```python
from build123d import *

# Parameters (mm, degrees)
BOSS_EXTRUDE1_DEPTH  = 7
BOSS_EXTRUDE2_DEPTH  = 60.3
SKETCH1_5_W          = 63.3
SKETCH1_5_H          = 5
BOSS_EXTRUDE3_DEPTH  = 60.3
SKETCH2_R            = 2.65
SKETCH2_R_2          = 3.5
CUT_EXTRUDE1_DEPTH   = 5
SKETCH2_3_R          = 19.05
CUT_EXTRUDE2_DEPTH   = 1.6
CUT_EXTRUDE3_DEPTH   = 5
BOSS_EXTRUDE6_DEPTH  = 5
BOSS_EXTRUDE10_DEPTH = 5
SKETCH15_R           = 3
SKETCH15_R_2         = 2
CUT_EXTRUDE7_DEPTH   = 5
SKETCH16_R           = 10
CUT_EXTRUDE8_DEPTH   = 5
SKETCH27_W           = 25
SKETCH27_H           = 87.5
CUT_EXTRUDE10_DEPTH  = 7
SKETCH33_R           = 3.5
BOSS_EXTRUDE18_DEPTH = 20


with BuildPart() as part:
    # Sketch1 → Boss-Extrude1 (new body)
    with BuildSketch(Plane(origin=(0, 0, 0), x_dir=(1, 0, 0), z_dir=(0, 1, 0))):
        Polygon((-1.592164976, 82.5), (61.707835024, 82.5), (86.707835024, 82.5), (86.707835024, -5), (61.707835024, -5), (-1.592164976, -5), (-26.592164976, -5), (-26.592164976, 82.5), align=None)
    extrude(amount=-BOSS_EXTRUDE1_DEPTH)

    # Sketch1<3> → Boss-Extrude2 (add)
    with BuildSketch(Plane(origin=(0, 0, 0), x_dir=(1, 0, 0), z_dir=(0, 1, 0))):
        Polygon((1.407835024, 0), (58.707835024, 0), (61.707835024, 0), (61.707835024, -5), (-1.592164976, -5), (-1.592164976, 0), align=None)
    extrude(amount=BOSS_EXTRUDE2_DEPTH)

    # Sketch1<5> → Boss-Extrude3 (add)
    with BuildSketch(Plane(origin=(0, 0, 0), x_dir=(1, 0, 0), z_dir=(0, 1, 0))):
        with Locations((30.057835024, 80)):
            Rectangle(SKETCH1_5_W, SKETCH1_5_H)
    extrude(amount=BOSS_EXTRUDE3_DEPTH)

    # Sketch2 → Cut-Extrude1 (cut)
    with BuildSketch(Plane(origin=(0, 0, 0), x_dir=(-1, 0, 0), z_dir=(0, 0, -1))):
        with Locations((-6.487835024, 52.22)):
            Circle(SKETCH2_R)
        with Locations((-53.627835024, 52.22)):
            Circle(SKETCH2_R)
        with Locations((-53.627835024, 5.08)):
            Circle(SKETCH2_R)
        with Locations((-6.487835024, 5.08)):
            Circle(SKETCH2_R)
        with Locations((-30.057835024, 28.65)):
            Circle(SKETCH2_R_2)
    extrude(amount=-CUT_EXTRUDE1_DEPTH, mode=Mode.SUBTRACT)

    # Sketch2<3> → Cut-Extrude2 (cut)
    with BuildSketch(Plane(origin=(0, 0, 0), x_dir=(-1, 0, 0), z_dir=(0, 0, -1))):
        with Locations((-30.057835024, 28.65)):
            Circle(SKETCH2_3_R)
    extrude(amount=-CUT_EXTRUDE2_DEPTH, mode=Mode.SUBTRACT)

    # Sketch4 → Cut-Extrude3 (cut)
    with BuildSketch(Plane.XY.offset(5)):
        Polygon((28.713159107, 31.881384638), (61.707835024, 45.611457374), (61.707835024, 38.029568262), (31.402510942, 25.418615362), align=None)
    extrude(amount=-CUT_EXTRUDE3_DEPTH, mode=Mode.SUBTRACT)

    # Sketch7 → Boss-Extrude6 (add)
    with BuildSketch(Plane(origin=(0, 0, -82.5), x_dir=(-1, 0, 0), z_dir=(0, 0, -1))):
        with BuildLine():
            Line((-61.707835024, 60.3), (-61.707835024, 98.3))
            ThreePointArc((-61.707835024, 98.3), (-30.057835024, 129.95), (1.592164976, 98.3))
            Line((1.592164976, 98.3), (1.592164976, 60.3))
            Line((1.592164976, 60.3), (-61.707835024, 60.3))
        make_face()
    extrude(amount=-BOSS_EXTRUDE6_DEPTH)

    # Sketch8 → Boss-Extrude10 (add)
    with BuildSketch(Plane.XY.offset(5)):
        with BuildLine():
            Line((-1.592164976, 60.3), (-1.592164976, 98.3))
            ThreePointArc((-1.592164976, 98.3), (30.057835024, 129.95), (61.707835024, 98.3))
            Line((61.707835024, 98.3), (61.707835024, 60.3))
            Line((61.707835024, 60.3), (-1.592164976, 60.3))
        make_face()
    extrude(amount=-BOSS_EXTRUDE10_DEPTH)

    # Sketch15 → Cut-Extrude7 (cut)
    with BuildSketch(Plane(origin=(0, 0, -82.5), x_dir=(-1, 0, 0), z_dir=(0, 0, -1))):
        with Locations((-30.057835024, 98.3)):
            Circle(SKETCH15_R)
        with Locations((-30.057835024, 105.8)):
            Circle(SKETCH15_R_2)
        with Locations((-22.557835024, 98.3)):
            Circle(SKETCH15_R_2)
        with Locations((-30.057835024, 90.8)):
            Circle(SKETCH15_R_2)
        with Locations((-37.557835024, 98.3)):
            Circle(SKETCH15_R_2)
    extrude(amount=-CUT_EXTRUDE7_DEPTH, mode=Mode.SUBTRACT)

    # Sketch16 → Cut-Extrude8 (cut)
    with BuildSketch(Plane.XY.offset(5)):
        with Locations((30.057835024, 98.3)):
            Circle(SKETCH16_R)
    extrude(amount=-CUT_EXTRUDE8_DEPTH, mode=Mode.SUBTRACT)

    # Sketch27 → Cut-Extrude10 (cut)
    with BuildSketch(Plane(origin=(0, 0, 0), x_dir=(1, 0, 0), z_dir=(0, 1, 0))):
        with Locations((74.207835024, 38.75)):
            Rectangle(SKETCH27_W, SKETCH27_H)
        with Locations((-14.092164976, 38.75)):
            Rectangle(SKETCH27_W, SKETCH27_H)
    extrude(amount=-CUT_EXTRUDE10_DEPTH, mode=Mode.SUBTRACT)

    # Sketch33 → Boss-Extrude18 (add)
    with BuildSketch(Plane.XY.offset(-77.5)):
        with Locations((30.057835024, 30.15)):
            Circle(SKETCH33_R)
    extrude(amount=-BOSS_EXTRUDE18_DEPTH)


solid = part.part
```
Check sheet for the modelled part. Datum: model origin and axes. Units: mm. A direction names the side the tool comes from. Round coordinates to 2 decimals unless told otherwise and drop trailing zeros. Loops run counter-clockwise (first coordinate to the right, second up) from the corner with the lowest first, then second, coordinate; pieces in that order, holes last. Notation, with made-up numbers: (-9, -37.5) -> (-3, -37.5) arc R19 ccw to (-3, -6.5) -> close; hole circle Ø4 at (-13, 49). An arc over 180 degrees is marked (long way). Write item = value, one per line. Start each with the question number.
1) Sectioned sample at A-A, the plane y = 5.08. Record the cut outline in (x, z).
2) Sectioned sample at D-D, the plane x = 17.5. Record the cut outline in (y, z).
3) Thickness scan on probe 1 along X at (y, z) = (98, -81); probe 2 along Z at (x, y) = (11, 47.5); probe 3 along Z at (x, y) = (21, 21). Record the ranges inside material, lowest first.
4) Sectioned sample at B-B, the plane y = 28.65. Record the cut outline in (x, z).
5) Gauge pin test, flat ends, axial feed: pin 1 Ø3 at (x, y) = (7.5, 52) entering from +Z; pin 2 Ø2.5 at (x, y) = (22.56, 98.3) entering from +Z; pin 3 Ø6.5 at (x, y) = (30.06, 90.8) entering from -Z; pin 4 Ø2 at (x, z) = (27.5, -28.5) entering from +Y. Record the tip position at first contact, or that the pin passes through.
6) Release check for a two-part mould opening along Y. For faces 6 (the flat face through (30, 66, -77.5)), 7 (the cylindrical face through (30.491, 103.848, -80.035)), 8 (the flat face through (31, 0, -39)), 9 (the flat face through (31, -7, -39)) record: released by +Y, released by -Y, zero draft, split by the parting line, or undercut.
7) Sectioned sample at C-C, the plane z = -86. Record the cut outline in (x, y).
8) Set-up check for faces 1 (the cylindrical face through (26.86, 27.23, 3.28)), 2 (the flat face through (31, 66, 0)), 3 (the cylindrical face through (33.396, 31.201, -89.895)), 4 (the cylindrical face through (12.788, 20.61, 0.789)), 5 (the flat face through (30, 30, -97.5)): record each of +Z, -Z, +X, -X, +Y, -Y from which the full face is reachable in a straight line by a thin tool's end or side.
Results are:
q1.outline = (-1.59, -82.5) -> (61.71, -82.5) -> (61.71, -77.5) -> (-1.59, -77.5) -> close; (-1.59, 0) -> (3.84, 0) -> (3.84, 5) -> (-1.59, 5) -> close; (9.14, 0) -> (50.98, 0) -> (50.98, 5) -> (9.14, 5) -> close; (56.28, 0) -> (61.71, 0) -> (61.71, 5) -> (56.28, 5) -> close
q2.outline = (-7, -82.5) -> (127.35, -82.5) -> (127.35, -77.5) -> (0, -77.5) -> (0, 0) -> (14.33, 0) -> (14.33, 1.6) -> (42.97, 1.6) -> (42.97, 0) -> (127.35, 0) -> (127.35, 5) -> (-7, 5) -> close
q3.probe_1 = -1.59 to 20.58, 24.54 to 27.07, 33.04 to 35.58, 39.54 to 61.71
q3.probe_2 = -82.5 to -77.5, 0 to 5
q3.probe_3 = -82.5 to -77.5, 1.6 to 5
q4.outline = (-1.59, -82.5) -> (26.9, -82.5) -> (26.9, -97.5) -> (33.22, -97.5) -> (33.22, -82.5) -> (61.71, -82.5) -> (61.71, -77.5) -> (-1.59, -77.5) -> close; (-1.59, 0) -> (11.01, 0) -> (11.01, 1.6) -> (26.56, 1.6) -> (26.56, 5) -> (-1.59, 5) -> close; (39.17, 1.6) -> (49.11, 1.6) -> (49.11, 0) -> (61.71, 0) -> (61.71, 5) -> (39.17, 5) -> close
q5.pin_1 = -77.5
q5.pin_2 = through
q5.pin_3 = -82.5
q5.pin_4 = 0
q6.face_6 = zero draft
q6.face_7 = undercut
q6.face_8 = released by +Y
q6.face_9 = released by -Y
q7.outline = circle Ø7 at (30.06, 30.15)
q8.face_1 = +Z
q8.face_2 = +X, -X, +Y
q8.face_3 = -Z
q8.face_4 = none
q8.face_5 = -Z, +X, -X, +Y, -Y
